Design review of the part built by this model. Coordinates are the model's own, in mm. Round coordinates to 2 decimals unless told otherwise and drop trailing zeros. Loops run counter-clockwise (first coordinate to the right, second up) from the corner with the lowest first, then second, coordinate; pieces in that order, holes last. Notation, with made-up numbers: (78, 89) -> (106, 89) arc R16 ccw to (106, 111) -> close; hole circle Ø10 at (-5.75, -35). An arc over 180 degrees is marked (long way). Answer as CSV lines item,"result". Start each with the question number.
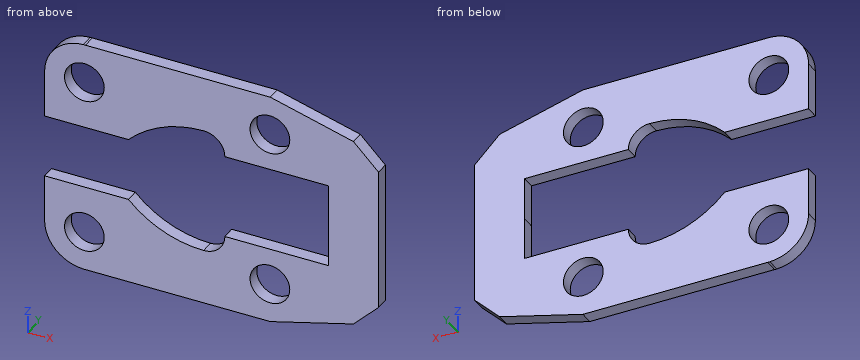
```python
from build123d import *

# Parameters (mm, degrees)
F0_R     = 9.525
F1_DEPTH = 6.35


with BuildPart() as f1:
    # F0 (on Front) → F1 (new body)
    with BuildSketch(Plane.XZ):
        with BuildLine():
            ThreePointArc((-44.203452, 57.142624), (-57.329882, 51.381651), (-62.723372, 38.1))
            Line((-62.723372, 38.1), (-62.723372, 15.24))
            Line((-62.723372, 15.24), (-22.559377, 15.24))
            ThreePointArc((-22.559377, 15.24), (-6.067452, 26.468514), (13.476628, 30.48))
            ThreePointArc((13.476628, 30.48), (20.660833, 27.504205), (23.636628, 20.32))
            Line((23.636628, 20.32), (73.318773, 20.32))
            Line((73.318773, 20.32), (73.420628, 0))
            Line((73.420628, 0), (73.318773, -20.32))
            Line((73.318773, -20.32), (23.636628, -20.32))
            ThreePointArc((23.636628, -20.32), (20.660833, -27.504205), (13.476628, -30.48))
            ThreePointArc((13.476628, -30.48), (-6.067452, -26.468514), (-22.559377, -15.24))
            Line((-22.559377, -15.24), (-62.723372, -15.24))
            Line((-62.723372, -15.24), (-62.723372, -38.1))
            ThreePointArc((-62.723372, -38.1), (-57.329882, -51.381651), (-44.203452, -57.142624))
            Line((-44.203452, -57.142624), (-43.143292, -57.142624))
            Line((-43.143292, -57.142624), (45.408478, -57.142624))
            Line((45.408478, -57.142624), (85.268794, -46.462084))
            Line((85.268794, -46.462084), (97.296628, -34.43425))
            Line((97.296628, -34.43425), (97.296628, 0))
            Line((97.296628, 0), (97.296628, 34.43425))
            Line((97.296628, 34.43425), (85.268794, 46.462084))
            Line((85.268794, 46.462084), (45.408478, 57.142624))
            Line((45.408478, 57.142624), (-43.143292, 57.142624))
            Line((-43.143292, 57.142624), (-44.203452, 57.142624))
        make_face()
        with Locations((-43.673372, -38.1)):
            Circle(F0_R, mode=Mode.SUBTRACT)
        with Locations((45.226628, -38.1)):
            Circle(F0_R, mode=Mode.SUBTRACT)
        with Locations((-43.673372, 38.1)):
            Circle(F0_R, mode=Mode.SUBTRACT)
        with Locations((45.226628, 38.1)):
            Circle(F0_R, mode=Mode.SUBTRACT)
        with BuildLine():
            ThreePointArc((-43.143292, 57.142624), (-43.673372, 57.15), (-44.203452, 57.142624))
            Line((-44.203452, 57.142624), (-43.143292, 57.142624))
        make_face()
        with BuildLine():
            ThreePointArc((-44.203452, -57.142624), (-43.673372, -57.15), (-43.143292, -57.142624))
            Line((-43.143292, -57.142624), (-44.203452, -57.142624))
        make_face()
    extrude(amount=F1_DEPTH)


solid = f1.part
```
Q1. Add section C-C, the plane z = 40. Give the boundary of the cut face in (x, y), and give its area (3 significant figures).
Q2. Add section B-B, the plane x = 71.5. Give the boundary of the cut face in (y, z).
Q3. For pin 1 Ø3 at (x, y) = (27.5, -1) entering from -Z; pin 2 Ø12 at (x, z) = (50.5, -37) entering from -Y; pin 3 Ø1.9 at (x, y) = (49.5, -3) entering from +Z, all flat-tipped, find the tip position at first contact; note any pin that passes through.
Q4. To check wall thickness, follow probe 1 along Z at (x, y) = (45, -5); probe 2 along Z at (x, y) = (-45.5, -4.75); probe 3 along X at (y, z) = (-6, -37). State the ranges of each line that lie inside material, in increasing order. Write a range as from..to.
Q5. Add section A-A, the plane y = -3.25. Give the boundary of the cut face in (x, z) (3 decimals).
Q6. Add section D-D, the plane x = -49.5. Give the boundary of the cut face in (y, z), and give its area (3 significant figures).
Worked answers:
1,outline,"(-62.63, -6.35) -> (-53.01, -6.35) -> (-53.01, 0) -> (-62.63, 0) -> close; (-34.34, -6.35) -> (35.89, -6.35) -> (35.89, 0) -> (-34.34, 0) -> close; (54.56, -6.35) -> (91.73, -6.35) -> (91.73, 0) -> (54.56, 0) -> close"
1,area,"743 mm^2"
2,outline,"(-6.35, -50.15) -> (0, -50.15) -> (0, -20.32) -> (-6.35, -20.32) -> close; (-6.35, 20.32) -> (0, 20.32) -> (0, 50.15) -> (-6.35, 50.15) -> close"
3,pin 1,"stops at z = -57.14"
3,pin 2,"stops at y = -6.35"
3,pin 3,"stops at z = 56.3"
4,probe 1,"z = -57.14..-47.62, -28.58..-20.32, 20.32..28.58, 47.62..57.14"
4,probe 2,"z = -57.06..-47.45, -28.75..-15.24, 15.24..28.75, 47.45..57.06"
4,probe 3,"x = -62.72..-53.13, -34.21..35.77, 54.69..94.73"
5,outline,"(-62.723, -38.1) arc R19.05 ccw to (-44.203, -57.143) arc R19.051 ccw to (-43.143, -57.143) -> (45.408, -57.143) -> (85.269, -46.462) -> (97.297, -34.434) -> (97.297, 34.434) -> (85.269, 46.462) -> (45.408, 57.143) -> (-43.143, 57.143) arc R19.051 ccw to (-44.203, 57.143) arc R19.05 ccw to (-62.723, 38.1) -> (-62.723, 15.24) -> (-22.559, 15.24) arc R50.8 cw to (13.477, 30.48) arc R10.16 cw to (23.637, 20.32) -> (73.319, 20.32) -> (73.421, 0) -> (73.319, -20.32) -> (23.637, -20.32) arc R10.16 cw to (13.477, -30.48) arc R50.8 cw to (-22.559, -15.24) -> (-62.723, -15.24) -> close; hole circle Ø19.05 at (-43.673, -38.1); hole circle Ø19.05 at (-43.673, 38.1); hole circle Ø19.05 at (45.227, -38.1); hole circle Ø19.05 at (45.227, 38.1)"
6,outline,"(-6.35, -56.24) -> (0, -56.24) -> (0, -45.63) -> (-6.35, -45.63) -> close; (-6.35, -30.57) -> (0, -30.57) -> (0, -15.24) -> (-6.35, -15.24) -> close; (-6.35, 15.24) -> (0, 15.24) -> (0, 30.57) -> (-6.35, 30.57) -> close; (-6.35, 45.63) -> (0, 45.63) -> (0, 56.24) -> (-6.35, 56.24) -> close"
6,area,"329 mm^2"
